Design review of the part built by this model. Coordinates are the model's own, in mm. Coordinates: 2 decimals unless noted, no trailing zeros. Write each loop counter-clockwise with the first axis right and the second up, starting at its lowest first coordinate (ties: lowest second). Pieces come first, ordered by that corner, then holes. Notation, with made-up numbers: (78.5, 7.25) - (117.5, 7.25) arc R19 cw to (117.5, 39.25) - close; hole circle Ø10 at (85, -4). An arc over 180 degrees is marked (long way). Answer as CSV lines item,"result". Start each with the question number.
Q1. We need section A-A (y = 256). Write out the cut boundary in (x, z), plus the area to 3 significant figures.
Q2. For line 1 along X through (y, z) = (322.5, -20); line 2 along Z through (x, y) = (-0.75, 335.5); line 3 along Z through (x, y) = (-11, 353), list the stretches that pass through material, from the lowest coordinate up. Write a range as [from, to].
Q3. Clearance check with flat-ended pins moving along their axes: pin 1 (4.5 mm diameter, centred on x = 9, y = 248.5, fed in from +Z); pin 2 (1.5 mm diameter, centred on y = 260, z = -17.5, fed in from +X); pin 3 (5 mm diameter, centred on x = 8, z = 1, fed in from +Y); pin 4 (8 mm diameter, centred on y = 204, z = -12, fed in from -X). State where each tip first meets the part, or that it passes through.
from build123d import *

# Parameters (mm, degrees)
F1_DEPTH = 500


with BuildPart() as f1:
    # F0 (on Front) → F1 (new body)
    with BuildSketch(Plane.XZ):
        with BuildLine():
            ThreePointArc((3.5355339059, -3.5355339059), (4.6193976626, -1.9134171618), (5, 0))
            ThreePointArc((5, 0), (-1.9134171618, 4.6193976626), (-3.5355339059, -3.5355339059))
            Line((-3.5355339059, -3.5355339059), (0, 0))
            Line((0, 0), (3.5355339059, -3.5355339059))
        make_face()
        with BuildLine():
            Line((0, 0), (-3.5355339059, -3.5355339059))
            ThreePointArc((-3.5355339059, -3.5355339059), (-1.9134171618, -4.6193976626), (0, -5))
            Line((0, -5), (0, 0))
        make_face()
        with BuildLine():
            ThreePointArc((0, -5), (-1.9134171618, -4.6193976626), (-3.5355339059, -3.5355339059))
            Line((-3.5355339059, -3.5355339059), (-6, -6))
            Line((-6, -6), (-6, -22))
            Line((-6, -22), (0, -22))
            Line((0, -22), (0, -5))
        make_face()
        with BuildLine():
            Line((6, -6), (3.5355339059, -3.5355339059))
            ThreePointArc((3.5355339059, -3.5355339059), (1.9134171618, -4.6193976626), (0, -5))
            Line((0, -5), (0, -22))
            Line((0, -22), (6, -22))
            Line((6, -22), (6, -6))
        make_face()
        with BuildLine():
            ThreePointArc((0, -5), (1.9134171618, -4.6193976626), (3.5355339059, -3.5355339059))
            Line((3.5355339059, -3.5355339059), (0, 0))
            Line((0, 0), (0, -5))
        make_face()
        Polygon((6, -22), (0, -22), (0, -26), (15, -26), (15, -22), align=None)
        Polygon((0, -26), (0, -22), (-6, -22), (-15, -22), (-15, -26), align=None)
    extrude(amount=-F1_DEPTH)


solid = f1.part
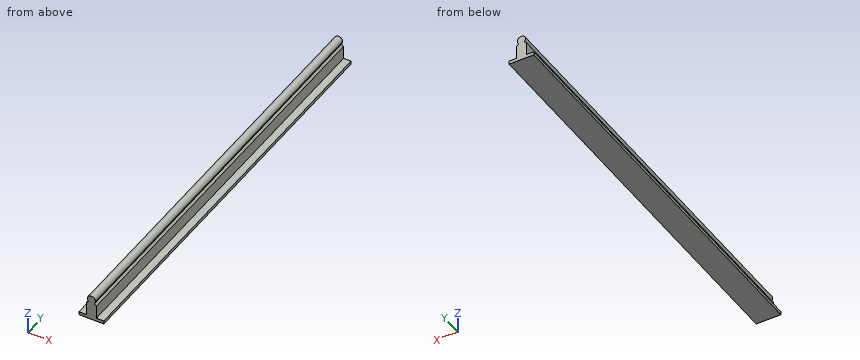
Results list:
1,outline,"(-15, -26) - (15, -26) - (15, -22) - (6, -22) - (6, -6) - (3.54, -3.54) arc R5 ccw (long way) to (-3.54, -3.54) - (-6, -6) - (-6, -22) - (-15, -22) - close"
1,area,"407 mm2"
2,line 1,"x = [-6, 6]"
2,line 2,"z = [-26, 4.94]"
2,line 3,"z = [-26, -22]"
3,pin 1,"stops at z = -22"
3,pin 2,"stops at x = 6"
3,pin 3,"passes through"
3,pin 4,"stops at x = -6"
